The listing builds one solid part. Answer for the finished solid, in the listing's coordinates (mm). Face numbers are marked on the shaded views. A direction names the side the tool comes from. Coordinates: 2 decimals unless noted, no trailing zeros. Loops run counter-clockwise (first coordinate to the right, second up) from the corner with the lowest first, then second, coordinate; pieces in that order, holes last. Notation, with made-up numbers: M 22,45 L 74,45 A20 ccw 74,77 Z; hole C 76.5,13 d10. An arc over 180 degrees is marked long. Return JSON: item names as keys, results as strings. Group by question number.
1. Which of the six approach directions +Z, -Z, +X, -X, +Y, -Y give full straight-line access (tool end or side, diameter ignored) to the marked faces 1, 2, 3, 4 and 5?
2. Straight lines are drawn through the part: L1, parallel to X at y = 48, z = 9.5; L2, parallel to Y at x = -96, z = 0. For each, find the intervals that lie inside material, in ascending order. Write a range as from..to.
3. Section A-A (y = 0) is taken. Write down the section's boundary in (x, z).
4. Given P1, Ø1, axis at x = -81.5, z = -95.5, coming from the -Y side; P2, Ø1.5, axis at y = 7.5, z = 25, coming from the -X side; P3, Ø20.5, axis at x = -278.5, y = -57.5, coming from the -Z side, each flat-ended and moving along its own axis, determine where each tip first touches the part or whether it passes through.
5. Section C-C (x = -232) is taken. Write down the section's boundary in (y, z).
6. Section B-B (z = -25.5) is taken. Write down the section's boundary in (x, y), then the cut area to 3 significant figures.
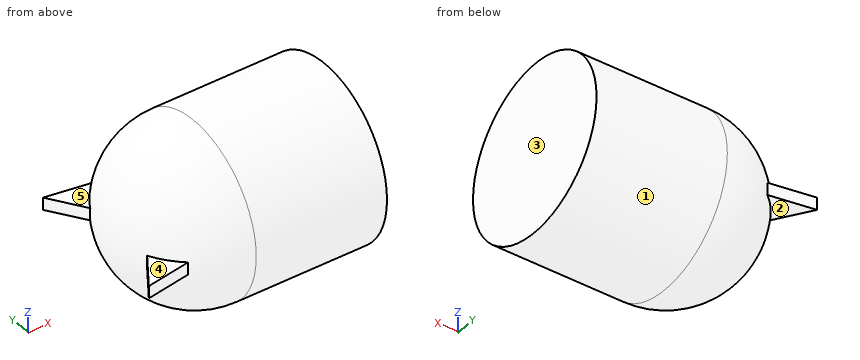
```python
from build123d import *

# Parameters (mm, degrees)
EXTRUDE_1_DEPTH      = 10
EXTRUDE_1_DEPTH_BACK = 10


with BuildPart() as part:
    # ｽｹｯﾁ2 → 回転-薄板1 (revolve)
    with BuildSketch(Plane.XY):
        with BuildLine():
            ThreePointArc((-327.5, 0), (-290.156114601, 90.156114601), (-200, 127.5))
            Line((-200, 127.5), (0, 127.5))
            Line((0, 127.5), (0, 0))
            Line((0, 0), (10, 0))
            Line((10, 0), (10, 137.5))
            Line((10, 137.5), (-200, 137.5))
            ThreePointArc((-200, 137.5), (-297.227182413, 97.227182413), (-337.5, 0))
            Line((-337.5, 0), (-327.5, 0))
        make_face()
    revolve(axis=Axis((0, 0, 0), (-1, 0, 0)))

    # ｽｹｯﾁ3 → ﾎﾞｽ - 押し出し1 (add, two sides: drawn at the far end of the back side and taken through both)
    with BuildSketch(Plane.XY.offset(-EXTRUDE_1_DEPTH_BACK)):
        Polygon((-302.60266968, 34.89733032), (-358.272990838, 117.779688618), (-239.232172231, 98.267827769), align=None)
        Polygon((-358.272990838, -117.779688618), (-239.232172231, -98.267827769), (-302.60266968, -34.89733032), align=None)
    extrude(amount=EXTRUDE_1_DEPTH + EXTRUDE_1_DEPTH_BACK)


solid = part.part
```
Worked out:
{
 "1": {"face 1": "+X, -X", "face 2": "-Z, -X, +Y", "face 3": "+Z, -Z, +X, +Y, -Y", "face 4": "+Z, -X, -Y", "face 5": "+Z, -X, +Y"},
 "2": {"L1": "-328.5..-317.74, -311.4..-289.5, 0..10", "L2": "-137.5..-127.5, 127.5..137.5"},
 "3": {"outline": "M -200,-137.5 L 10,-137.5 L 10,137.5 L -200,137.5 A137.5 ccw Z; hole M -200,-127.5 L 0,-127.5 L 0,127.5 L -200,127.5 A127.5 ccw Z"},
 "4": {"P1": "y = -99.4", "P2": "x = -335.14", "P3": "z = -106.43"},
 "5": {"outline": "C 0,0 d267.45; hole C 0,0 d246.84"},
 "6": {"outline": "M -200,-135.11 L 10,-135.11 L 10,135.11 L -200,135.11 A135.11 ccw Z; hole M -200,-124.92 L 0,-124.92 L 0,124.92 L -200,124.92 A124.92 ccw Z", "area": "10,900 mm^2"}
}
